Verification items for the finished model (mm, model axes). Face numbers are marked on the shaded views. A direction names the side the tool comes from. Round coordinates to 2 decimals unless told otherwise and drop trailing zeros. Loops run counter-clockwise (first coordinate to the right, second up) from the corner with the lowest first, then second, coordinate; pieces in that order, holes last. Notation, with made-up numbers: (27.25, -25) - (33.25, -25) arc R10 ccw to (33.25, -9) - close; hole circle Ø4 at (-30, -6.5). An arc over 180 degrees is marked (long way). Use CSV: the item, a comma, the result in double quotes.
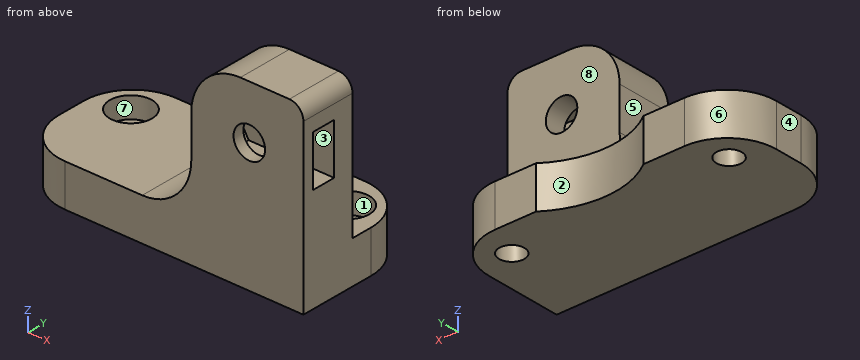
```python
from build123d import *

# Parameters (mm, degrees)
BOSS_EXTRUDE2_DEPTH  = 41
SKETCH3_R            = 1.8
SKETCH3_R_2          = 13
CUT_EXTRUDE1_DEPTH   = 47.701177715
M4_CLEARANCE_HOLE1_D = 4.5
SKETCH6_R            = 3
CUT_EXTRUDE2_DEPTH   = 3
CUT_EXTRUDE3_START   = -6.4
SKETCH7_R            = 2.25
CUT_EXTRUDE3_DEPTH   = 3.4
FILLET3_R            = 2
SKETCH9_W            = 25
SKETCH9_H            = 20
CUT_EXTRUDE5_DEPTH   = 47.701177715
FILLET5_R            = 7


with BuildPart() as part:
    # Sketch2 → Boss-Extrude2 (new body)
    with BuildSketch(Plane(origin=(0, 0, 0), x_dir=(0, 0, -1), z_dir=(1, 0, 0))):
        Polygon((0, 0), (0, 10), (6, 10), (6, -8), (-20, -8), (-20, 0), align=None)
    extrude(amount=BOSS_EXTRUDE2_DEPTH)

    # Sketch3 → Cut-Extrude1 (cut, through all)
    with BuildSketch(Plane.XY):
        with Locations((5, 5)):
            Circle(SKETCH3_R)
        with Locations((36, 5)):
            Circle(SKETCH3_R)
        with Locations((20.5, 20.5)):
            Circle(SKETCH3_R_2)
    extrude(amount=-CUT_EXTRUDE1_DEPTH, mode=Mode.SUBTRACT)

    # M4 Clearance Hole1 (through all)
    with Locations(Plane(origin=(33.28379107, 0, 12.4), x_dir=(0, 0, 1), z_dir=(0, 1, 0))):
        with Locations((0, 0)):
            Hole(M4_CLEARANCE_HOLE1_D / 2)

    # Sketch6 → Cut-Extrude2 (cut)
    with BuildSketch(Plane.XY):
        with Locations((5, 5)):
            Circle(SKETCH6_R)
        with Locations((36, 5)):
            Circle(SKETCH6_R)
    extrude(amount=-CUT_EXTRUDE2_DEPTH, mode=Mode.SUBTRACT)

    # Sketch7 → Cut-Extrude3 (cut)
    with BuildSketch(Plane(origin=(0, 0, 0), x_dir=(1, 0, 0), z_dir=(0, 1, 0)).offset(CUT_EXTRUDE3_START)):
        with Locations(Location((33.28379107, -12.4, 0), (0, 0, 270))):
            Circle(SKETCH7_R)
        Polygon((26.726869132, -12.4), (28.805330101, -16), (32.962252039, -16), (35.040713008, -12.4), (32.962252039, -8.8), (28.805330101, -8.8), align=None)
        with BuildLine():
            Line((33.772715521, -14.596236071), (32.962252039, -16))
            Line((32.962252039, -16), (41, -16))
            Line((41, -16), (41, -8.8))
            Line((41, -8.8), (32.962252039, -8.8))
            Line((32.962252039, -8.8), (33.772715521, -10.203763929))
            ThreePointArc((33.772715521, -10.203763929), (35.039151434, -10.992445386), (35.53379107, -12.4))
            ThreePointArc((35.53379107, -12.4), (35.039151434, -13.807554614), (33.772715521, -14.596236071))
        make_face()
    extrude(amount=CUT_EXTRUDE3_DEPTH, mode=Mode.SUBTRACT)

    # Fillet3
    fillet3_edges = [part.edges().sort_by_distance(p)[0] for p in [
        (41, -4, 20),
    ]]
    fillet(fillet3_edges, radius=FILLET3_R)

    # Sketch9 → Cut-Extrude5 (cut, through all)
    with BuildSketch(Plane(origin=(0, 0, 0), x_dir=(1, 0, 0), z_dir=(0, 1, 0))):
        with Locations((12.5, -10)):
            Rectangle(SKETCH9_W, SKETCH9_H)
    extrude(amount=-CUT_EXTRUDE5_DEPTH, mode=Mode.SUBTRACT)

    # Fillet5
    fillet5_edges = [part.edges().sort_by_distance(p)[0] for p in [
        (41, 10, -3),
        (0, -8, -3),
        (0, 10, -3),
        (25, -4, 0),
        (25, -4, 20),
    ]]
    fillet(fillet5_edges, radius=FILLET5_R)


solid = part.part
```
1) Cross-section at A-A, the plane z = -2. Record the cut outline in (x, y), then the cut area to 3 significant figures.
Returned:
outline,"(0, -1) arc R7 ccw to (7, -8) - (41, -8) - (41, 3) arc R7 ccw to (34, 10) - (28.16, 10) arc R13 cw to (12.84, 10) - (7, 10) arc R7 ccw to (0, 3) - close; hole circle Ø6 at (5, 5); hole circle Ø6 at (36, 5)"
area,"624 mm²"
2) Gauge pin test, flat ends, axial feed: pin 1 Ø4.5 at (x, y) = (36, 5) entering from -Z; pin 2 Ø4 at (y, z) = (0.5, 4) entering from -X; pin 3 Ø1.8 at (x, y) = (36, 5) entering from +Z; pin 4 Ø8 at (x, y) = (5, 5) entering from +Z. Record the tip position at first contact, or that the pin passes through.
Returned:
pin 1,"stops at z = -6"
pin 2,"stops at x = 22.96"
pin 3,"passes through"
pin 4,"stops at z = 0"
3) Cross-section at C-C, the plane y = 4. Record the cut outline in (x, z), then the cut area to 3 significant figures.
Returned:
outline,"(0.07, -6) - (3.5, -6) - (3.5, -3) - (2.17, -3) - (2.17, 0) - (0.07, 0) - close; (6.5, -6) - (34.5, -6) - (34.5, -3) - (33.17, -3) - (33.17, 0) - (7.83, 0) - (7.83, -3) - (6.5, -3) - close; (37.5, -6) - (40.93, -6) - (40.93, 0) - (38.83, 0) - (38.83, -3) - (37.5, -3) - close"
area,"193 mm²"
4) Thickness scan on probe 1 along Y at (x, z) = (34.5, 15.75); probe 2 along Z at (x, y) = (33, -5.25); probe 3 along Z at (x, y) = (15, -2). Record the ranges inside material, lowest first. Write a range as [from, to].
Returned:
probe 1,"y = [-8, -6.4], [-3, 0]"
probe 2,"z = [-6, 8.8], [16, 20]"
probe 3,"z = [-6, 0]"
5) Access from +Z, -Z, +X, -X, +Y, -Y to the whole of each face (thin tool, end or side, straight path). Record for the marked faces 5, 6, 7 and 8.
Returned:
face 5,"+Z, -X, +Y, -Y"
face 6,"+Z, -Z, -X, +Y"
face 7,"+Z"
face 8,"+Z, +X, -X, +Y"
6) Cross-section at B-B, the plane x = 36. Record the cut outline in (y, z).
Returned:
outline,"(-8, -6) - (3.2, -6) - (3.2, -3) - (2, -3) - (2, 0) - (0, 0) - (0, 20) - (-8, 20) - close; (6.8, -6) - (9.71, -6) - (9.71, 0) - (8, 0) - (8, -3) - (6.8, -3) - close; hole (-6.4, 8.8) - (-3, 8.8) - (-3, 16) - (-6.4, 16) - close"
7) Mould release check, pull along X, two halves, no side actions. Record for the marked faces 1, 2, 3 and 4: +X half, -X half, draft (parallel to the pull), parting line (faces both ways), or undercut.
Returned:
face 1,"undercut"
face 2,"undercut"
face 3,"draft"
face 4,"-X half"
8) Cross-section at D-D, the plane x = 5. Record the cut outline in (y, z), then the cut area to 3 significant figures.
Returned:
outline,"(-7.71, -6) - (3.2, -6) - (3.2, -3) - (2, -3) - (2, 0) - (-7.71, 0) - close; (6.8, -6) - (9.71, -6) - (9.71, 0) - (8, 0) - (8, -3) - (6.8, -3) - close"
area,"75.7 mm²"
